Can you work these out from the model? Positions are in its coordinate system, mm. Give positions to 0.01 mm unless a question says otherwise; leave off trailing zeros. Write each loop counter-clockwise with the first axis right and the second up, starting at its lowest first coordinate (ties: lowest second). Pieces come first, ordered by that corner, then holes. Notation, with made-up numbers: (-34.5, 80.5) -> (-17.5, 80.5) arc R19 cw to (-17.5, 106.5) -> close; hole circle Ø1 at (18.5, 22). An arc over 180 degrees is marked (long way). One line per item, written item: value.
from build123d import *

# Parameters (mm, degrees)
CROQUIS1_R              = 7.5
CROQUIS1_R_2            = 10
SALIENTE_EXTRUIR1_DEPTH = 10
CROQUIS2_R              = 10
SALIENTE_EXTRUIR2_DEPTH = 75
CROQUIS3_R              = 5
SALIENTE_EXTRUIR3_DEPTH = 16
CROQUIS4_R              = 4
SALIENTE_EXTRUIR4_DEPTH = 22


with BuildPart() as part:
    # Croquis1 → Saliente-Extruir1 (new body)
    with BuildSketch(Plane.XY):
        with BuildLine():
            Line((-20, 0), (-20, 60))
            ThreePointArc((-20, 60), (-13.639967201, 74.627074032), (1.395129475, 79.951281005))
            Line((1.395129475, 79.951281005), (340.566906563, 56.234079932))
            ThreePointArc((340.566906563, 56.234079932), (359.123058094, 34.887669452), (337.776647613, 16.331517922))
            Line((337.776647613, 16.331517922), (30.697564737, 37.804579202))
            ThreePointArc((30.697564737, 37.804579202), (23.180016399, 35.142475715), (20, 27.828938699))
            Line((20, 27.828938699), (20, 0))
            ThreePointArc((20, 0), (0, -20), (-20, 0))
        make_face()
        Circle(CROQUIS1_R, mode=Mode.SUBTRACT)
        with Locations((339.171777088, 36.282798927)):
            Circle(CROQUIS1_R_2, mode=Mode.SUBTRACT)
    extrude(amount=SALIENTE_EXTRUIR1_DEPTH)

    # Croquis2 → Saliente-Extruir2 (add)
    with BuildSketch(Plane(origin=(0, 0, 0), x_dir=(-1, 0, 0), z_dir=(0, 0, -1))):
        with Locations((0, 60)):
            Circle(CROQUIS2_R)
    extrude(amount=SALIENTE_EXTRUIR2_DEPTH)

    # Croquis3 → Saliente-Extruir3 (add)
    with BuildSketch(Plane(origin=(0, 0, -75), x_dir=(-1, 0, 0), z_dir=(0, 0, -1))):
        with Locations((0, 60)):
            Circle(CROQUIS3_R)
    extrude(amount=SALIENTE_EXTRUIR3_DEPTH)

    # Croquis4 → Saliente-Extruir4 (add)
    with BuildSketch(Plane.XY.offset(10)):
        with Locations((0, 60)):
            Circle(CROQUIS4_R)
    extrude(amount=SALIENTE_EXTRUIR4_DEPTH)


solid = part.part
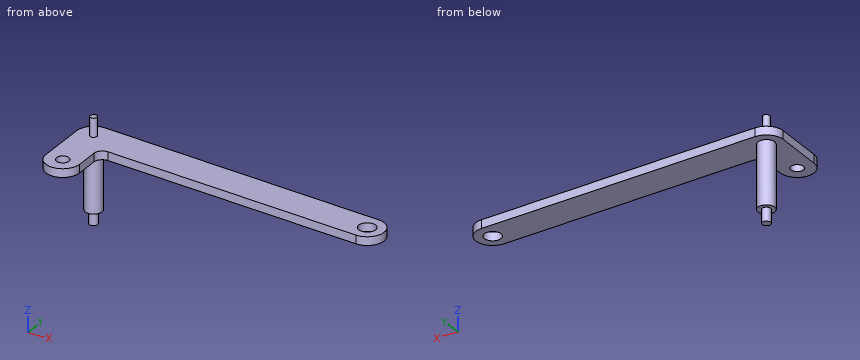
1) If we section it at A-A (z = -78.5): Write out the boundary of the cut face in (x, y), and give its area (3 significant figures).
Answer list:
outline: circle Ø10 at (0, 60)
area: 78.5 mm^2
2) If we section it at D-D (z = 15): Write out the boundary of the cut face in (x, y).
Answer list:
outline: circle Ø8 at (0, 60)
3) If we section it at C-C (x = 300.5): Write out the boundary of the cut face in (y, z).
Answer list:
outline: (18.94, 0) -> (59.04, 0) -> (59.04, 10) -> (18.94, 10) -> close
4) If we section it at B-B (y = 73.5): Write out the boundary of the cut face in (x, z).
Answer list:
outline: (-14.76, 0) -> (93.65, 0) -> (93.65, 10) -> (-14.76, 10) -> close
5) Will these pins go through, and if not, where does the flat tip stop? pin 1 (3 mm diameter, centred on y = 60, z = -8, fed in from -X); pin 2 (5 mm diameter, centred on x = 146.5, y = 52.5, fed in from +Z); pin 3 (3 mm diameter, centred on y = 7.5, z = 4.5, fed in from +X).
Answer list:
pin 1: stops at x = -10
pin 2: stops at z = 10
pin 3: stops at x = 20
6) I need wall thicknesses on L1, parallel to Z at x = 147, y = 38; L2, parallel to X at y = 67, z = -47.5; L3, parallel to X at y = 55.5, z = -79. Which ranges of each line are inside material? Lowest first, please.
Answer list:
L1: z = 0 to 10
L2: x = -7.14 to 7.14
L3: x = -2.18 to 2.18
